Verification items for the finished model (mm, model axes). Face numbers are marked on the shaded views. A direction names the side the tool comes from. Coordinates: 2 decimals unless noted, no trailing zeros. Write each loop counter-clockwise with the first axis right and the second up, starting at its lowest first coordinate (ties: lowest second). Pieces come first, ordered by that corner, then holes. Notation, with made-up numbers: M 68,33 L 92,33 A21 ccw 92,71 Z; hole C 46,21 d10. An arc over 180 degrees is marked long. One line per item, written item: value.
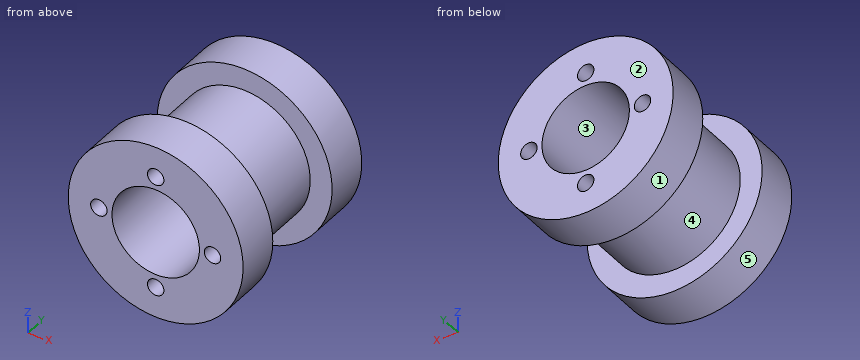
```python
from build123d import *

# Parameters (mm, degrees)
F0_R     = 12.7
F1_DEPTH = 6.35
F2_R     = 9.525
F3_DEPTH = 12.7
F4_R     = 12.7
F5_DEPTH = 6.35
F7_D     = 12.7
F8_D     = 2.3876


with BuildPart() as f1:
    # F0 (on Front) → F1 (new body)
    with BuildSketch(Plane.XZ):
        Circle(F0_R)
    extrude(amount=F1_DEPTH)

    # F2 (on face) → F3 (join)
    with BuildSketch(Plane(origin=(0, 0, 0), x_dir=(-1, 0, 0), z_dir=(0, 1, 0))):
        Circle(F2_R)
    extrude(amount=F3_DEPTH)

    # F4 (on face) → F5 (join)
    with BuildSketch(Plane(origin=(0, 12.7, 0), x_dir=(-1, 0, 0), z_dir=(0, 1, 0))):
        Circle(F4_R)
    extrude(amount=F5_DEPTH)

    # F7 (through all)
    with Locations(Plane.XZ.offset(6.35)):
        with Locations((0, 0)):
            Hole(F7_D / 2)

    # F8 (through all)
    with Locations(Plane.XZ.offset(6.35)):
        with Locations((0, 8.255), (-8.2519316698, 0.2250526986), (0, -8.255), (8.255, 0)):
            Hole(F8_D / 2)


solid = f1.part
```
Item 1: Cross-section at D-D, the plane y = 6.5. Enter the section's corners in (x, z) (3 decimals), and give its area (3 significant figures).
The answers:
outline: C 0,0 d19.05; hole C -8.252,0.225 d2.388; hole C 0,0 d12.7; hole C 0,-8.255 d2.388; hole C 0,8.255 d2.388; hole C 8.255,0 d2.388
area: 140 mm²
Item 2: Scan lines: line 1 (Z direction, x = 0, y = -0.75); line 2 (Y direction, x = -7.5, z = 6.5); line 3 (X direction, y = 12.25, z = 8.25). Record each from-to range of solid material in increasing order.
The answers:
line 1: z = -12.7 to -9.45, -7.06 to -6.35, 6.35 to 7.06, 9.45 to 12.7
line 2: y = -6.35 to 0, 12.7 to 19.05
line 3: x = -4.76 to -1.19, 1.19 to 4.76
Item 3: Cross-section at C-C, the plane x = -8.25. Enter the section's corners in (y, z), and give its area (3 significant figures).
The answers:
outline: M -6.35,-9.66 L 0,-9.66 L 0,-4.76 L 12.7,-4.76 L 12.7,-9.66 L 19.05,-9.66 L 19.05,-0.97 L -6.35,-0.97 Z; M -6.35,1.42 L 19.05,1.42 L 19.05,9.66 L 12.7,9.66 L 12.7,4.76 L 0,4.76 L 0,9.66 L -6.35,9.66 Z
area: 306 mm²
Item 4: Go/stop test with flat-tipped pins: P1, Ø1, axis at y = 3, z = 7.5, coming from the +X side; P2, Ø2.5, axis at x = -8.25, z = 0.23, coming from the +Y side; P3, Ø5, axis at x = 7, y = -0.5, coming from the +Z side; P4, Ø1.9, axis at x = 8.255, z = 0, coming from the -Y side. Record where each tip stops, or that it passes through.
The answers:
P1: stops at x = 6.46
P2: stops at y = 19.05
P3: stops at z = 11.88
P4: passes through
Item 5: Access from +Z, -Z, +X, -X, +Y, -Y to the whole of each face (thin tool, end or side, straight path). Record for the marked faces 4 and 5.
The answers:
face 4: none
face 5: +Y, -Y
Item 6: Cross-section at A-A, the plane x = 0. Enter the section's corners in (y, z) (3 decimals).
The answers:
outline: M -6.35,-12.7 L 0,-12.7 L 0,-9.525 L 12.7,-9.525 L 12.7,-12.7 L 19.05,-12.7 L 19.05,-9.449 L -6.35,-9.449 Z; M -6.35,-7.061 L 19.05,-7.061 L 19.05,-6.35 L -6.35,-6.35 Z; M -6.35,6.35 L 19.05,6.35 L 19.05,7.061 L -6.35,7.061 Z; M -6.35,9.449 L 19.05,9.449 L 19.05,12.7 L 12.7,12.7 L 12.7,9.525 L 0,9.525 L 0,12.7 L -6.35,12.7 Z
Item 7: Cross-section at B-B, the plane z = 4. Enter the section's corners in (x, y).
The answers:
outline: M -12.05,-6.35 L -4.93,-6.35 L -4.93,19.05 L -12.05,19.05 L -12.05,12.7 L -8.64,12.7 L -8.64,0 L -12.05,0 Z; M 4.93,-6.35 L 12.05,-6.35 L 12.05,0 L 8.64,0 L 8.64,12.7 L 12.05,12.7 L 12.05,19.05 L 4.93,19.05 Z
Item 8: Draft check along X on the marked faces 1, 2 and 3. Enter one of: released by +X, released by -X, zero draft, split by the parting line, or undercut.
The answers:
face 1: split by the parting line
face 2: zero draft
face 3: undercut
